from build123d import *

# Parameters (mm, degrees)
F0_R      = 41.275
F0_R_2    = 40.005
F1_DEPTH  = 3.175
F3_DEPTH  = 4.445
F5_DEPTH  = 6.351
F6_R      = 3.175
F8_D      = 4.4
F9_R      = 41.275
F9_R_2    = 40.005
F10_DEPTH = 1.5875
F11_SIZE  = 1.26999


# Not quite as in the source:
# - a fillet or chamfer is up to 0.001 mm smaller than in the source, because OpenCascade refuses the exact size


with BuildPart() as f1:
    # F0 (on Front) → F1 (new body, symmetric)
    with BuildSketch(Plane.XZ):
        Circle(F0_R)
        Circle(F0_R_2, mode=Mode.SUBTRACT)
        Circle(F0_R_2)
        Polygon((-7.3323484187, 0), (-3.6661742094, 6.35), (3.6661742094, 6.35), (7.3323484187, 0), (3.6661742094, -6.35), (-3.6661742094, -6.35), align=None, mode=Mode.SUBTRACT)
        Polygon((3.6661742094, 6.35), (-3.6661742094, 6.35), (-7.3323484187, 0), (-3.6661742094, -6.35), (3.6661742094, -6.35), (7.3323484187, 0), align=None)
    extrude(amount=F1_DEPTH, both=True)

    # F2 (on face) → F3 (cut)
    with BuildSketch(Plane.XZ.offset(3.175)):
        Polygon((7.1846849266, 0.1208628901), (3.4876721301, 6.2825511097), (-3.6970127965, 6.1616882196), (-7.1846849266, -0.1208628901), (-3.4876721301, -6.2825511097), (3.6970127965, -6.1616882196), align=None)
    extrude(amount=-F3_DEPTH, mode=Mode.SUBTRACT)

    # F4 (on face) → F5 (cut, through all)
    with BuildSketch(Plane.XZ.offset(3.175)):
        with BuildLine():
            ThreePointArc((-35.1952724098, -5.08), (-25.144717139, -25.144717139), (-5.08, -35.1952724098))
            Line((-5.08, -35.1952724098), (-5.08, -11.6397422652))
            ThreePointArc((-5.08, -11.6397422652), (-8.9802561211, -8.9802561211), (-11.6397422652, -5.08))
            Line((-11.6397422652, -5.08), (-35.1952724098, -5.08))
        make_face()
        with BuildLine():
            Line((-5.08, 11.6397422652), (-5.08, 35.1952724098))
            ThreePointArc((-5.08, 35.1952724098), (-25.144717139, 25.144717139), (-35.1952724098, 5.08))
            Line((-35.1952724098, 5.08), (-11.6397422652, 5.08))
            ThreePointArc((-11.6397422652, 5.08), (-8.9802561211, 8.9802561211), (-5.08, 11.6397422652))
        make_face()
        with BuildLine():
            Line((11.6397422652, 5.08), (35.1952724098, 5.08))
            ThreePointArc((35.1952724098, 5.08), (25.144717139, 25.144717139), (5.08, 35.1952724098))
            Line((5.08, 35.1952724098), (5.08, 11.6397422652))
            ThreePointArc((5.08, 11.6397422652), (8.9802561211, 8.9802561211), (11.6397422652, 5.08))
        make_face()
        with BuildLine():
            ThreePointArc((5.08, -35.1952724098), (25.144717139, -25.144717139), (35.1952724098, -5.08))
            Line((35.1952724098, -5.08), (11.6397422652, -5.08))
            ThreePointArc((11.6397422652, -5.08), (8.9802561211, -8.9802561211), (5.08, -11.6397422652))
            Line((5.08, -11.6397422652), (5.08, -35.1952724098))
        make_face()
    extrude(amount=-F5_DEPTH, mode=Mode.SUBTRACT)

    # F6
    f6_edges = [f1.edges().sort_by_distance(p)[0] for p in [
        (-35.195272, 0, -5.08),
        (-11.639742, 0, -5.08),
        (-5.08, 0, -35.195272),
        (-5.08, 0, -11.639742),
        (5.08, 0, -35.195272),
        (5.08, 0, -11.639742),
        (35.195272, 0, -5.08),
        (11.639742, 0, -5.08),
        (-5.08, 0, 35.195272),
        (-5.08, 0, 11.639742),
        (-35.195272, 0, 5.08),
        (-11.639742, 0, 5.08),
        (35.195272, 0, 5.08),
        (11.639742, 0, 5.08),
        (5.08, 0, 35.195272),
        (5.08, 0, 11.639742),
    ]]
    fillet(f6_edges, radius=F6_R)

    # F8 (through all)
    with Locations(Plane.XZ.offset(-1.27)):
        with Locations((0, 0)):
            Hole(F8_D / 2)

    # F9 (on Front) → F10 (cut, symmetric)
    with BuildSketch(Plane.XZ):
        Circle(F9_R)
        Circle(F9_R_2, mode=Mode.SUBTRACT)
    extrude(amount=F10_DEPTH, both=True, mode=Mode.SUBTRACT)

    # F11 (size 1.27 in the source; OpenCascade refuses exactly that, so slightly less here)
    f11_edges = [f1.edges().sort_by_distance(p)[0] for p in [
        (-40.005, 1.5875, 0),
        (-40.005, -1.5875, 0),
    ]]
    chamfer(f11_edges, length=F11_SIZE)


solid = f1.part
Geometry: final body of the model. Coordinates: model frame, mm. A direction names the side the tool comes from. Coordinates: 2 decimals unless noted, no trailing zeros.
(1) First-contact query: pin 1 (3 mm diameter, centred on x = 24, y = 0, fed in from -Z); pin 2 (4 mm diameter, centred on x = 2.5, z = 2.5, fed in from -Y); pin 3 (3 mm diameter, centred on x = -6, y = 2.5, fed in from -Z). Flat tips, straight axial feed; report the tip coordinate or a pass-through.
(2) Section query B-B (z = -15). State how many separate pieces and enclosed holes the cut face has, plus the area to 3 significant figures.
(3) Access query for faces 1 (the face through (5.36, -0.98, 3.16)), 2 (the face through (-25.33, -0.04, -24.96)), 3 (the face through (-1, 3.175, -9)). Directions: +Z, -Z, +X, -X, +Y, -Y. A direction counts if a zero-diameter tool reaches every point of the face in a straight line with its end or side. Return the directions, or none.
(4) Draft query along X for faces 4 (the face through (5.5, 0.04, -11.98)), 5 (the face through (-1, -3.175, -9)), 6 (the face through (23, 0, -5.08)), 7 (the face through (-8.948, -2.392, -40.293)). Return one class per face: pulls with the +X half, pulls with the -X half, needs draft (parallel to the pull), parting line crosses it, or undercut.
(5) Material intervals for probe 1 along Z at (x, y) = (0, 1.8) (3 decimals); probe 2 along Z at (x, y) = (-9, -1.25); probe 3 along Z at (x, y) = (-26, -1.75), sorted ascending.
Solution:
1. pin 1: stops at z = -33.75
1. pin 2: stops at y = 1.27
1. pin 3: stops at z = -41.03
2. separate pieces: 3
2. enclosed holes: 0
2. area: 138 mm2
3. face 1: -Y
3. face 2: +Y, -Y
3. face 3: +Z, -Z, +X, -X, +Y
4. face 4: undercut
4. face 5: needs draft
4. face 6: undercut
4. face 7: parting line crosses it
5. probe 1: z = -41.275 to -2.2, 2.2 to 41.275
5. probe 2: z = -39.94 to -34.4, -8.96 to 8.96, 34.4 to 39.94
5. probe 3: z = -32.06 to -24.26, -5.08 to 5.08, 24.26 to 32.06
